Could you check a few things on this drawing? It's one solid part, dimensions in mm from its lowest x, y, z. Give positions to 0.01 mm unless a question says otherwise; leave off trailing zeros. Order: outer loops, then holes, each group sorted by start corner. A loop starts at its lowest first (then second) coordinate and runs counter-clockwise, first axis right, second up.
(1) Imagine slicing it at C-C, the plane x = 69. Write out the boundary of the cut face in (y, z), then the cut area to 3 significant figures.
(2) Imagine slicing it at B-B, the plane y = 1.6. Write out the boundary of the cut face in (x, z), then the cut area to 3 significant figures.
(3) If I drill on probe 1 along Z at (x, y) = (54, 4.55), over which ranges is the centre line in solid material (lowest first)?
(4) Imagine slicing it at A-A, the plane z = 11. Write out the boundary of the cut face in (x, y).
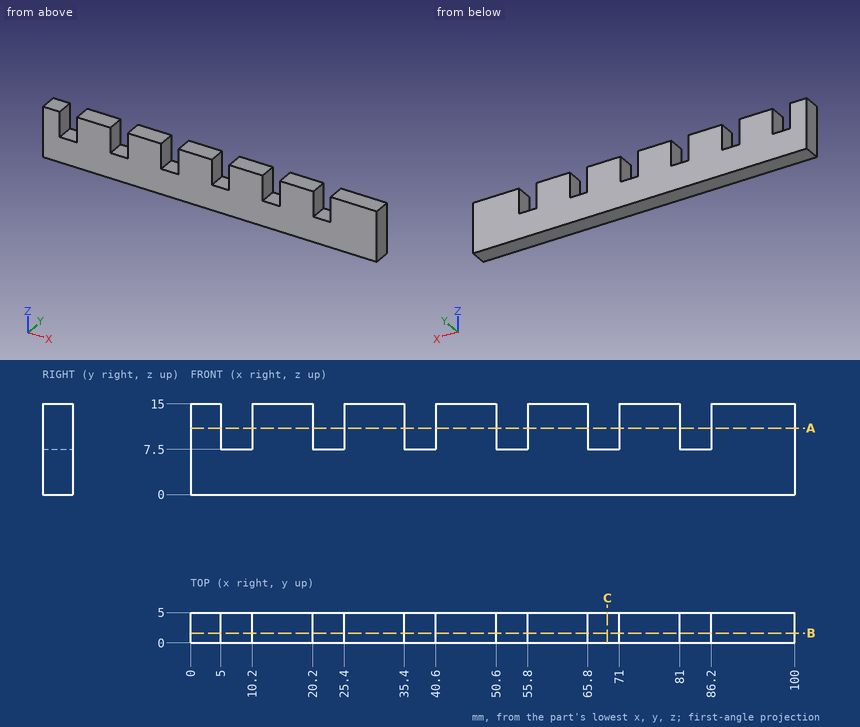
Answer block:
1. outline: (0, 0) - (5, 0) - (5, 7.5) - (0, 7.5) - close
1. area: 37.5 mm2
2. outline: (0, 0) - (100, 0) - (100, 15) - (86.2, 15) - (86.2, 7.5) - (81, 7.5) - (81, 15) - (71, 15) - (71, 7.5) - (65.8, 7.5) - (65.8, 15) - (55.8, 15) - (55.8, 7.5) - (50.6, 7.5) - (50.6, 15) - (40.6, 15) - (40.6, 7.5) - (35.4, 7.5) - (35.4, 15) - (25.4, 15) - (25.4, 7.5) - (20.2, 7.5) - (20.2, 15) - (10.2, 15) - (10.2, 7.5) - (5, 7.5) - (5, 15) - (0, 15) - close
2. area: 1,270 mm2
3. probe 1: z = 0 to 7.5
4. outline: (0, 0) - (5, 0) - (5, 5) - (0, 5) - close; (10.2, 0) - (20.2, 0) - (20.2, 5) - (10.2, 5) - close; (25.4, 0) - (35.4, 0) - (35.4, 5) - (25.4, 5) - close; (40.6, 0) - (50.6, 0) - (50.6, 5) - (40.6, 5) - close; (55.8, 0) - (65.8, 0) - (65.8, 5) - (55.8, 5) - close; (71, 0) - (81, 0) - (81, 5) - (71, 5) - close; (86.2, 0) - (100, 0) - (100, 5) - (86.2, 5) - close
